Check sheet for the modelled part. Datum: model origin and axes. Units: mm. A direction names the side the tool comes from. Coordinates: 2 decimals unless noted, no trailing zeros. Loops run counter-clockwise (first coordinate to the right, second up) from the corner with the lowest first, then second, coordinate; pieces in that order, holes last. Notation, with made-up numbers: (1.25, 6) - (31.25, 6) arc R30 cw to (31.25, 45) - close; hole circle Ø5 at (65.5, 43.25). An arc over 180 degrees is marked (long way). Write each question's results on one line, items separated by ' | '. Start each with the question number.
1. Cross-section at A-A (y = 30). Record the cut outline in (x, z), and give its area (3 significant figures).
2. Tool access check on faces 1 (the face through (0, -12, -27.095)), 2 (the face through (8.932, -17, -21)), 3 (the face through (23.47, -9.86, -6.97)), 4 (the face through (8.2, 113.97, 5.23)). Record the directions out of +Z, -Z, +X, -X, +Y, -Y that give a thin tool (end or side, any length) a straight path to the whole face; none if there is none.
3. Thickness scan on line 1 (Y direction, x = -24, z = 20.5); line 2 (Y direction, x = 5, z = -29); line 3 (X direction, y = -4.5, z = -4). Record the ranges inside material, lowest first. Write a range as [from, to].
4. Draft check along Y on faces 5 (the face through (15.96, -9.86, -9.12)), 6 (the face through (30.639, 3.192, -18.705)), 7 (the face through (0, -14, -14.617)), 8 (the face through (-27.477, -16.136, -15.54)). Enter one of: released by +Y, released by -Y, zero draft, split by the parting line, or undercut.
5. Gauge pin test, flat ends, axial feed: P1, Ø2.5, axis at x = -1.5, z = -28, coming from the +Y side; P2, Ø3, axis at y = 2, z = 24, coming from the -X side; P3, Ø8, axis at y = 17.5, z = -3.5, coming from the -X side; P4, Ø1.5, axis at x = 1.5, z = 4.5, coming from the -Y side. Record the tip position at first contact, or that the pin passes through.
```python
from build123d import *

# Parameters (mm, degrees)
SKETCH_2_R               = 31.689767185
EXTRUDE_1_DEPTH          = 10
SKETCH_3_W               = 11.398540158
SKETCH_3_H               = 11.018588819
EXTRUDE_2_DEPTH          = 20
CUT_EXTRUDE_1_DEPTH      = 20
SKETCH_6_R               = 20
EXTRUDE_3_DEPTH          = 4
PATTERN_CIRCULAR_2_COUNT = 3
EXTRUDE_4_DEPTH          = 4
EXTRUDE_5_DEPTH          = 17.8
PATTERN_CIRCULAR_3_COUNT = 3
SKETCH_9_R               = 5.625050713
EXTRUDE_6_DEPTH          = 19
SKETCH_10_R              = 1.630795406
EXTRUDE_7_DEPTH          = 100
PATTERN_CIRCULAR_4_COUNT = 3
SKETCH_11_R              = 31.689767185
EXTRUDE_8_DEPTH          = 2
SKETCH_12_R              = 9.724605512
EXTRUDE_9_DEPTH          = 4


with BuildPart() as part:
    # 草图2 → 凸台-拉伸1 (new body)
    with BuildSketch(Plane(origin=(0, 0, 0), x_dir=(1, 0, 0), z_dir=(0, 1, 0))):
        with Locations(Location((0, 0, 0), (0, 0, 270))):
            Circle(SKETCH_2_R)
    extrude(amount=EXTRUDE_1_DEPTH)

    # 草图3 → 凸台-拉伸2 (add)
    with BuildSketch(Plane.XZ):
        with Locations((0, 23.889440414)):
            Rectangle(SKETCH_3_W, SKETCH_3_H)
    extrude_2 = extrude(amount=EXTRUDE_2_DEPTH)

    # 草图4 → 切除-拉伸1 (cut)
    with BuildSketch(Plane(origin=(5.699270079, 0, 0), x_dir=(0, 0, -1), z_dir=(1, 0, 0))):
        Polygon((-29.398734823, -10), (-26.056890095, -20), (-29.398734823, -20), align=None)
    cut_extrude_1 = extrude(amount=-CUT_EXTRUDE_1_DEPTH, mode=Mode.SUBTRACT)

    # 草图6 → 凸台-拉伸3 (add)
    with BuildSketch(Plane(origin=(0, -9.842221306, 29.451462012), x_dir=(1, 0, 0), z_dir=(0, -0.316954203171244, 0.9484408432222232))):
        with Locations(Location((0, -5.578767415, 0), (0, 0, 270))):
            Circle(SKETCH_6_R)
    extrude_3 = extrude(amount=EXTRUDE_3_DEPTH)

    # 阵列(圆周)2: 凸台-拉伸2, 切除-拉伸1, 凸台-拉伸3 ×3 about axis
    pattern_circular_2_axis = Axis((0, 0, 0), (0, 1, 0))
    add([extrude_2.rotate(pattern_circular_2_axis, i * 360 / PATTERN_CIRCULAR_2_COUNT) for i in range(1, PATTERN_CIRCULAR_2_COUNT)])
    add([cut_extrude_1.rotate(pattern_circular_2_axis, i * 360 / PATTERN_CIRCULAR_2_COUNT) for i in range(1, PATTERN_CIRCULAR_2_COUNT)], mode=Mode.SUBTRACT)
    add([extrude_3.rotate(pattern_circular_2_axis, i * 360 / PATTERN_CIRCULAR_2_COUNT) for i in range(1, PATTERN_CIRCULAR_2_COUNT)])

    # 草图7 → 凸台-拉伸4 (add)
    with BuildSketch(Plane.XZ):
        with BuildLine():
            Line((-4.433868769, 7.679685983), (0, 10.23958131))
            Line((0, 10.23958131), (-19.030711532, 21.226967736))
            Line((-19.030711532, 21.226967736), (-27.898449071, 5.86759577))
            Line((-27.898449071, 5.86759577), (-8.867737539, -5.119790655))
            Line((-8.867737539, -5.119790655), (-8.867737539, 0))
            ThreePointArc((-8.867737539, 0), (-7.679685983, 4.433868769), (-4.433868769, 7.679685983))
        make_face()
        with BuildLine():
            ThreePointArc((4.433868769, 7.679685983), (7.679685983, 4.433868769), (8.867737539, 0))
            Line((8.867737539, 0), (8.867737539, -5.119790655))
            Line((8.867737539, -5.119790655), (27.898449071, 5.86759577))
            Line((27.898449071, 5.86759577), (19.030711532, 21.226967736))
            Line((19.030711532, 21.226967736), (0, 10.23958131))
            Line((0, 10.23958131), (4.433868769, 7.679685983))
        make_face()
        with BuildLine():
            Line((8.867737539, -27.094563507), (8.867737539, -5.119790655))
            Line((8.867737539, -5.119790655), (4.433868769, -7.679685983))
            ThreePointArc((4.433868769, -7.679685983), (0, -8.867737539), (-4.433868769, -7.679685983))
            Line((-4.433868769, -7.679685983), (-8.867737539, -5.119790655))
            Line((-8.867737539, -5.119790655), (-8.867737539, -27.094563507))
            Line((-8.867737539, -27.094563507), (8.867737539, -27.094563507))
        make_face()
        with BuildLine():
            ThreePointArc((4.433868769, -7.679685983), (7.679685983, -4.433868769), (8.867737539, 0))
            ThreePointArc((8.867737539, 0), (7.679685983, 4.433868769), (4.433868769, 7.679685983))
            ThreePointArc((4.433868769, 7.679685983), (0, 8.867737539), (-4.433868769, 7.679685983))
            ThreePointArc((-4.433868769, 7.679685983), (-7.679685983, 4.433868769), (-8.867737539, 0))
            ThreePointArc((-8.867737539, 0), (-7.679685983, -4.433868769), (-4.433868769, -7.679685983))
            ThreePointArc((-4.433868769, -7.679685983), (0, -8.867737539), (4.433868769, -7.679685983))
        make_face()
        with BuildLine():
            Line((8.867737539, -5.119790655), (8.867737539, 0))
            ThreePointArc((8.867737539, 0), (7.679685983, -4.433868769), (4.433868769, -7.679685983))
            Line((4.433868769, -7.679685983), (8.867737539, -5.119790655))
        make_face()
        with BuildLine():
            Line((-8.867737539, -5.119790655), (-4.433868769, -7.679685983))
            ThreePointArc((-4.433868769, -7.679685983), (-7.679685983, -4.433868769), (-8.867737539, 0))
            Line((-8.867737539, 0), (-8.867737539, -5.119790655))
        make_face()
        with BuildLine():
            ThreePointArc((-4.433868769, 7.679685983), (0, 8.867737539), (4.433868769, 7.679685983))
            Line((4.433868769, 7.679685983), (0, 10.23958131))
            Line((0, 10.23958131), (-4.433868769, 7.679685983))
        make_face()
    extrude(amount=EXTRUDE_4_DEPTH)

    # 草图8 → 凸台-拉伸5 (add)
    with BuildSketch(Plane(origin=(4.433868769, 0, -7.679685983), x_dir=(-0.8660254037844431, 0, -0.499999999999992), z_dir=(0.49999999999999206, 0, -0.8660254037844433))):
        with BuildLine():
            Line((-30.427113752, -29.482756554), (-30.427113752, -23.325905307))
            Line((-30.427113752, -23.325905307), (-27.094563507, -23.325905307))
            Line((-27.094563507, -23.325905307), (-27.094563507, -4))
            Line((-27.094563507, -4), (-14.617014317, -4))
            Line((-14.617014317, -4), (-14.617014317, -23.325905307))
            Line((-14.617014317, -23.325905307), (-11.847477178, -23.325905307))
            Line((-11.847477178, -23.325905307), (-11.847477178, -24.665032542))
            ThreePointArc((-11.847477178, -24.665032542), (-21.274112807, -26.546256084), (-30.427113752, -29.482756554))
        make_face()
    extrude_5 = extrude(amount=-EXTRUDE_5_DEPTH)

    # 阵列(圆周)3: 凸台-拉伸5 ×3 about axis
    pattern_circular_3_axis = Axis((0, 0, 0), (0, 1, 0))
    for i in range(1, PATTERN_CIRCULAR_3_COUNT):
        add(extrude_5.rotate(pattern_circular_3_axis, i * 360 / PATTERN_CIRCULAR_3_COUNT))

    # 草图9 → 凸台-拉伸6 (add)
    with BuildSketch(Plane.XZ.offset(4)):
        with Locations(Location((0, 0, 0), (0, 0, 270))):
            Circle(SKETCH_9_R)
    extrude(amount=EXTRUDE_6_DEPTH)

    # 草图10 → 凸台-拉伸7 (add)
    with BuildSketch(Plane(origin=(0, 10, 0), x_dir=(1, 0, 0), z_dir=(0, 1, 0))):
        with Locations(Location((0, -28.081418828, 0), (0, 0, 270))):
            Circle(SKETCH_10_R)
    extrude_7 = extrude(amount=EXTRUDE_7_DEPTH)

    # 阵列(圆周)4: 凸台-拉伸7 ×3 about axis
    pattern_circular_4_axis = Axis((0, 0, 0), (0, 1, 0))
    for i in range(1, PATTERN_CIRCULAR_4_COUNT):
        add(extrude_7.rotate(pattern_circular_4_axis, i * 360 / PATTERN_CIRCULAR_4_COUNT))

    # 草图11 → 凸台-拉伸8 (add)
    with BuildSketch(Plane(origin=(0, 110, 0), x_dir=(1, 0, 0), z_dir=(0, 1, 0))):
        with Locations(Location((0, 0, 0), (0, 0, 270))):
            Circle(SKETCH_11_R)
    extrude(amount=EXTRUDE_8_DEPTH)

    # 草图12 → 凸台-拉伸9 (add)
    with BuildSketch(Plane(origin=(0, 112, 0), x_dir=(1, 0, 0), z_dir=(0, 1, 0))):
        with Locations(Location((0, 0, 0), (0, 0, 270))):
            Circle(SKETCH_12_R)
    extrude(amount=EXTRUDE_9_DEPTH)


solid = part.part
```
Established:
1) outline: circle Ø3.26 at (-24.32, -14.04); circle Ø3.26 at (0, 28.08); circle Ø3.26 at (24.32, -14.04) | area: 25.1 mm^2
2) face 1: -Z | face 2: -Z, -Y | face 3: none | face 4: +Y
3) line 1: [0, 10], [110, 112] | line 2: [-28.95, -23.33], [0, 10], [110, 112] | line 3: [-38.24, -33.76], [-3.95, 3.95], [33.76, 38.24]
4) face 5: zero draft | face 6: split by the parting line | face 7: undercut | face 8: released by -Y
5) P1: y = 112 | P2: x = -22.32 | P3: through | P4: y = -23
